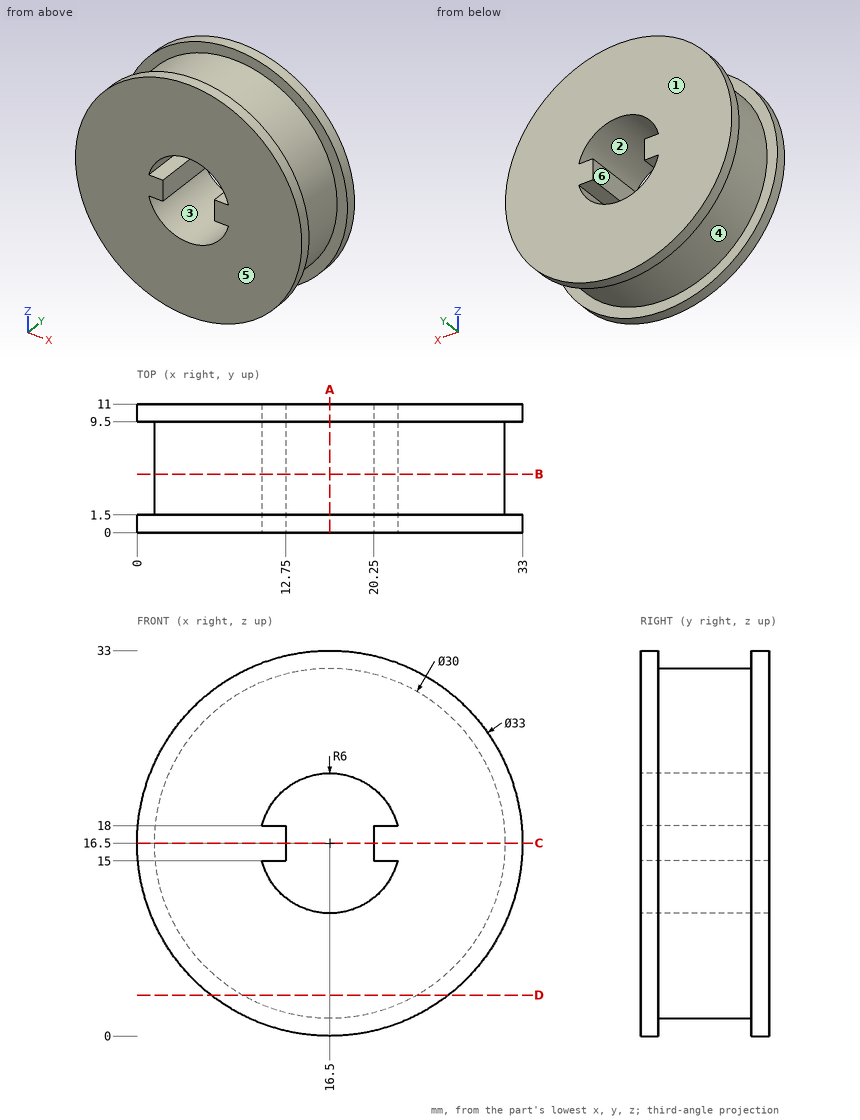
Geometry check sheet. Reference: drawing and pictorial views, mm from the part's lowest x, y, z. A direction names the side the tool comes from. Give positions to 0.01 mm unless a question says otherwise; leave off trailing zeros. Order: outer loops, then holes, each group sorted by start corner. A loop starts at its lowest first (then second) coordinate and runs counter-clockwise, first axis right, second up. Notation, with made-up numbers: M 35.25,63 L 41.25,63 A20 cw 41.25,95 Z; hole C 40.25,38 d8. An arc over 180 degrees is marked long. Return JSON: item names as keys, results as strings. Group by question number.
1) Mould release check, pull along Z, two halves, no side actions. Record for the marked faces 1, 2, 3 and 4: pulls with the +Z half, pulls with the -Z half, needs draft (parallel to the pull), parting line crosses it, or undercut.
2) Section check B-B on y = 5. Record the cut outline in (x, z), and give its area (3 significant figures).
3) Scan lines: line 1 (X direction, y = 7.25, z = 17); line 2 (Y direction, x = 6.5, z = 29); line 3 (Z direction, x = 20.5, y = 4.75). Record each from-to range of solid material in increasing order.
4) Section check D-D on z = 3.5. Record the cut outline in (x, y).
5) Go/stop test with flat-tipped pins: pin 1 Ø2 at (x, y) = (3.5, 2) entering from -Z; pin 2 Ø1 at (y, z) = (3, 16.5) entering from -X; pin 3 Ø1.6 at (x, y) = (21, 8) entering from +Z. Record where each tip stops, or that it passes through.
6) Access from +Z, -Z, +X, -X, +Y, -Y to the whole of each face (thin tool, end or side, straight path). Record for the marked faces 5 and 6.
7) Section check A-A on x = 16.5. Record the cut outline in (y, z), and give its area (3 significant figures).
8) Section check C-C on z = 16.5. Record the cut outline in (x, y), and give its area (4 significant figures).
Answer block:
{
 "1": {"face 1": "needs draft", "face 2": "undercut", "face 3": "undercut", "face 4": "parting line crosses it"},
 "2": {"outline": "C 16.5,16.5 d30; hole M 10.69,15 A6 ccw 22.31,15 L 20.25,15 L 20.25,18 L 22.31,18 A6 ccw 10.69,18 L 12.75,18 L 12.75,15 Z", "area": "607 mm^2"},
 "3": {"line 1": "x = 1.51 to 12.75, 20.25 to 31.49", "line 2": "y = 0 to 1.5, 9.5 to 11", "line 3": "z = 2.04 to 12.03, 15 to 18, 20.97 to 30.96"},
 "4": {"outline": "M 6.34,0 L 26.66,0 L 26.66,1.5 L 23.98,1.5 L 23.98,9.5 L 26.66,9.5 L 26.66,11 L 6.34,11 L 6.34,9.5 L 9.02,9.5 L 9.02,1.5 L 6.34,1.5 Z"},
 "5": {"pin 1": "stops at z = 5.32", "pin 2": "stops at x = 1.5", "pin 3": "stops at z = 31.04"},
 "6": {"face 5": "+Z, -Z, +X, -X, -Y", "face 6": "+Y, -Y"},
 "7": {"outline": "M 0,0 L 1.5,0 L 1.5,1.5 L 9.5,1.5 L 9.5,0 L 11,0 L 11,10.5 L 0,10.5 Z; M 0,22.5 L 11,22.5 L 11,33 L 9.5,33 L 9.5,31.5 L 1.5,31.5 L 1.5,33 L 0,33 Z", "area": "207 mm^2"},
 "8": {"outline": "M 0,0 L 12.75,0 L 12.75,11 L 0,11 L 0,9.5 L 1.5,9.5 L 1.5,1.5 L 0,1.5 Z; M 20.25,0 L 33,0 L 33,1.5 L 31.5,1.5 L 31.5,9.5 L 33,9.5 L 33,11 L 20.25,11 Z", "area": "256.5 mm^2"}
}
